from build123d import *


with BuildPart() as part:
    # Sketch1 → Revolve1 (revolve)
    with BuildSketch(Plane.XY, mode=Mode.PRIVATE) as revolve1_sk:
        with BuildLine():
            Line((8.763, 5.9563), (7.62, 4.3434))
            Line((7.62, 4.3434), (7.62, -4.3434))
            Line((7.62, -4.3434), (21.43125, -4.3434))
            Line((21.43125, -4.3434), (21.43125, -0.635))
            Line((21.43125, -0.635), (17.4625, -0.635))
            Line((17.4625, -0.635), (17.4625, 0.635))
            Line((17.4625, 0.635), (20.79625, 0.635))
            Line((20.79625, 0.635), (20.79625, 1.778))
            Line((20.79625, 1.778), (17.1196, 5.9563))
            ThreePointArc((17.1196, 5.9563), (12.9413, 10.1346), (8.763, 5.9563))
        make_face()
    revolve(revolve1_sk.sketch.rotate(Axis((0, 10.1346, 0), (0, -1, 0)), 90), axis=Axis((0, 10.1346, 0), (0, -1, 0)))


solid = part.part
Source: CAD feature listing. Evaluate the final solid. Frame: model axes, mm. A direction names the side the tool comes from. Give positions to 0.01 mm unless a question says otherwise; leave off trailing zeros. Write each loop counter-clockwise with the first axis right and the second up, starting at its lowest first coordinate (ties: lowest second). Pieces come first, ordered by that corner, then holes. Notation, with made-up numbers: (60, 68) -> (80, 68) arc R27 cw to (80, 86) -> close; hole circle Ø6 at (56, -4.5). An arc over 180 degrees is marked (long way). Write item = value, one per line.
Q1. Cut plane B-B on z = 0. Return loops of the section in (x, y) (1 decimal).
Here are the results:
outline = (-21.4, -4.3) -> (-7.6, -4.3) -> (-7.6, 4.3) -> (-8.8, 6) arc R4.2 ccw to (-17.1, 6) -> (-20.8, 1.8) -> (-20.8, 0.6) -> (-17.5, 0.6) -> (-17.5, -0.6) -> (-21.4, -0.6) -> close; (7.6, -4.3) -> (21.4, -4.3) -> (21.4, -0.6) -> (17.5, -0.6) -> (17.5, 0.6) -> (20.8, 0.6) -> (20.8, 1.8) -> (17.1, 6) arc R4.2 ccw to (8.8, 6) -> (7.6, 4.3) -> close
Q2. First-contact query: pin 1 (1 mm diameter, centred on x = -10.5, z = -15, fed in from +Y); pin 2 (5 mm diameter, centred on x = -12.5, y = -1, fed in from -Z); pin 3 (12 mm diameter, centred on x = 0, z = 0, fed in from +Y); pin 4 (8 mm diameter, centred on y = 4.5, z = -8, fed in from -X). Flat tips, straight axial feed; report the tip coordinate or a pass-through.
Here are the results:
pin_1 = 5.17
pin_2 = -18.96
pin_3 = through
pin_4 = -20.17
Q3. Cut plane A-A on x = 0. Return loops of the section in (y, z) (1 decimal), then the cut area to 3 significant figures.
Here are the results:
outline = (-4.3, -21.4) -> (-0.6, -21.4) -> (-0.6, -17.5) -> (0.6, -17.5) -> (0.6, -20.8) -> (1.8, -20.8) -> (6, -17.1) arc R4.2 ccw to (6, -8.8) -> (4.3, -7.6) -> (-4.3, -7.6) -> close; (-4.3, 7.6) -> (4.3, 7.6) -> (6, 8.8) arc R4.2 ccw to (6, 17.1) -> (1.8, 20.8) -> (0.6, 20.8) -> (0.6, 17.5) -> (-0.6, 17.5) -> (-0.6, 21.4) -> (-4.3, 21.4) -> close
area = 305 mm²
Q4. Reachability of faces 1 (the face through (0, -0.635, -18)), 2 (the face through (9, -4.343, 0)), 3 (the face through (-20.62, 1.21, -2.71)) from +Z, -Z, +X, -X, +Y, -Y: full face, straight path, thin tool, end or side. Return the list, or none.
Here are the results:
face_1 = none
face_2 = +Z, -Z, +X, -X, -Y
face_3 = +Y
Q5. Mould query, pull axis X, two halves, no side actions, for faces 4 (the face through (-7.555, -0.061, -0.992)), 5 (the face through (17, 0, -4)), 6 (the face through (-17, 0.635, 5)). Classes: +X half, -X half, draft (parallel to the pull), parting line (faces both ways), or undercut.
Here are the results:
face_4 = undercut
face_5 = parting line
face_6 = draft
Q6. Line query: line 1 (X direction, y = -1, z = 0); line 2 (X direction, y = 1.5, z = 0); line 3 (Y direction, x = -13.5, z = 16) (3 decimals). Output: solid intervals per line, ascending. Write a range as from..to.
Here are the results:
line_1 = -21.43..-7.62, 7.62..21.43
line_2 = -20.8..-7.62, 7.62..20.8
line_3 = -4.343..-0.635
Q7. Cut plane C-C on y = 7.5. Return loops of the section in (x, z), then the cut area to 3 significant figures.
Here are the results:
outline = circle Ø33.65 at (0, 0); hole circle Ø18.12 at (0, 0)
area = 631 mm²
